The listing builds one solid part. Answer for the finished solid, in the listing's coordinates (mm). Face numbers are marked on the shaded views. A direction names the side the tool comes from. Give positions to 0.01 mm unless a question says otherwise; leave off trailing zeros. Write each loop counter-clockwise with the first axis right and the second up, starting at its lowest first coordinate (ties: lowest second). Pieces come first, ordered by that corner, then holes. Notation, with made-up numbers: (58.25, -26) - (104.25, -26) arc R37 cw to (104.25, 10) - close; hole circle Ø3 at (29.25, -22). An arc over 180 degrees is marked (long way). One line per question, with ' | ' between items. Start each with the question number.
1. A cutting plane is placed at D-D (x = -35). Determine the outline of the cut face in (y, z), then the cut area to 3 significant figures.
2. Given P1, Ø6, axis at x = 17, y = -1, coming from the +Z side; P2, Ø6, axis at x = -12, z = 6, coming from the +Y side; P3, Ø1, axis at y = 2, z = 4, coming from the +X side, each flat-ended and moving along its own axis, determine where each tip first touches the part or whether it passes through.
3. A cutting plane is placed at B-B (z = 9). Determine the outline of the cut face in (x, y), then the cut area to 3 significant figures.
4. A cutting plane is placed at C-C (x = 12). Determine the outline of the cut face in (y, z).
5. Find the intervals of material crossed by L1, parallel to Y at x = 0, z = 7.75; L2, parallel to X at y = -1.5, z = 1.5; L3, parallel to X at y = -0.5, z = 5.25, in increasing order. Write a range as from..to.
6. For the marked faces 1 and 2, determine the directions among +Z, -Z, +X, -X, +Y, -Y from which every point of the face is accessible in a straight line to the end or side of a thin tool.
7. A cutting plane is placed at A-A (x = 0). Determine the outline of the cut face in (y, z).
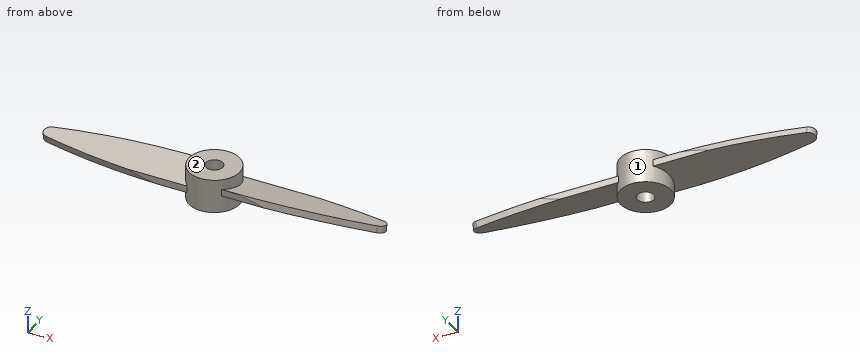
Autodesk Inventor part; units mm, degrees
ref_plane "Work Plane1" through (0, 7.5, 0) normal (0, 1, 0) x (-1, 0, 0)
ref_plane "Work Plane2" through (-7.5, 0, 0) normal (1, 0, 0) x (0, 1, 0)
ref_plane "Work Plane3" through (7.5, 0, 0) normal (1, 0, 0) x (0, 1, 0)
sketch "Sketch - Propeller Connecter" plane through (0, 0, 0) normal (0, 0, 1) x (1, 0, 0)
  circle A0 centre (0, 0) radius 7.5
  circle A1 centre (0, 0) radius 2.5
  dimension "d0" = 15
  dimension "d1" = 5
extrude "Extrusion1" add sketch "Sketch - Propeller Connecter" along normal blind 10
ref_plane "Work Plane1" through (0, 7.5, 0) normal (0, 1, 0) x (-1, 0, 0)
ref_plane "Work Plane2" through (-7.5, 0, 0) normal (1, 0, 0) x (0, 1, 0)
sketch "Sketch3" plane through (-7.5, 0, 0) normal (1, 0, 0) x (0, 1, 0)
  line L0 (7.5, 10) -> (-7.5, 10)
  line L1 (7.5, 10) -> (7.5, 0)
  line L2 (7.5, 0) -> (7.5, 10)
  line L3 (-7.5, 0) -> (7.5, 0)
  line L4 (-7.5, 10) -> (-7.5, 0)
  line L5 (-7.5, 0) -> (-7.5, 10)
  line L6 (5.5, 7) -> (-5.5, 5)
  line L7 (5.5, 5) -> (-5.5, 3)
  line L8 (5.5, 5) -> (5.5, 7)
  line L9 (-5.5, 3) -> (-5.5, 5)
  point P0 (0, 0)
  point P1 (0, 5)
  dimension "d27" = 5
  dimension "d28" = 3
  dimension "d29" = 3
  dimension "d30" = 5
  dimension "d32" = 2
  dimension "d33" = 2
  dimension "d34" = 2
  dimension "d35" = 2
sketch3d "3D Sketch2"
ref_plane "Work Plane3" through (7.5, 0, 0) normal (1, 0, 0) x (0, 1, 0)
sketch "Sketch4" plane through (7.5, 0, 0) normal (1, 0, 0) x (0, 1, 0)
  line L0 (5.5, 5) -> (-5.5, 7)
  line L1 (5.5, 3) -> (-5.5, 5)
  line L2 (5.5, 3) -> (5.5, 5)
  line L3 (-5.5, 5) -> (-5.5, 7)
  line L4 (7.5, 10) -> (-7.5, 10)
  line L5 (-7.5, 0) -> (7.5, 0)
  line L6 (-7.5, 0) -> (-7.5, 10)
  line L7 (7.5, 0) -> (7.5, 10)
  point P0 (0, 0)
  point P1 (0, 5)
  dimension "d38" = 3
  dimension "d39" = 5
  dimension "d40" = 3
  dimension "d42" = 5
  dimension "d43" = 2
  dimension "d44" = 2
  dimension "d45" = 2
  dimension "d46" = 2
sketch3d "3D Sketch3"
extrude "Extrusion2" add sketch "Sketch4" against normal blind 5 contours L2 L1 L3 L0
extrude "Extrusion3" add sketch "Sketch4" along normal blind 50 contours L2 L1 L3 L0
extrude "Extrusion4" add sketch "Sketch3" along normal blind 5 contours L8 L7 L9 L6
extrude "Extrusion5" add sketch "Sketch3" against normal blind 50 contours L8 L7 L9 L6
sketch "Sketch8" plane through (-5.099, -5.5, 3) normal (0, 0.1788854, -0.9838699) x (-1, 0, 0)
  line L0 (52.401, 0) -> (0, 0)
  line L1 (52.401, 11.1803) -> (52.401, 0)
  arc A0 (2.3083, 0) -> (52.401, 5.5902) centre (5.3498, 199.9769) ccw
  line L2 (52.401, 5.5902) -> (52.401, 0)
  line L3 (52.401, 0) -> (8.3914, 0)
  point P0 (-5.099, 4.8746)
  dimension "d59" = 200
extrude "Extrusion6" cut sketch "Sketch8" against normal blind 30 contours L0 A0 L1
sketch "Sketch15" plane through (57.5, 5.5, 3) normal (0, -0.1788854, -0.9838699) x (-1, 0, 0)
  line L0 (52.401, -0.3578) -> (52.401, 0)
  arc A0 (52.401, 0) -> (-0.7421, -4.8746) centre (43.9347, -199.8207) ccw
  line L1 (-0.7421, -4.8746) -> (-0.7421, 0)
  line L2 (-0.7421, 0) -> (35.4685, 0)
  point P0 (57.5, -4.8746)
  dimension "d67" = 200
extrude "Extrusion7" cut sketch "Sketch15" against normal blind 30
sketch "Sketch16" plane through (-57.5, 5.5, 7) normal (0, -0.1788854, 0.9838699) x (1, 0, 0)
  line L0 (52.401, -0.3578) -> (52.401, 0)
  line L1 (0, -5.9479) -> (0, 0)
  arc A0 (52.401, 0) -> (0, -5.9479) centre (48.5604, -199.9631) ccw
  line L2 (0, 0) -> (44.7198, 0)
  line L3 (52.401, 0) -> (0, 0)
  point P0 (57.5, -6.6635)
  dimension "d70" = 200
extrude "Extrusion8" cut sketch "Sketch16" against normal blind 30 contours L1 L2 A0
sketch "Sketch17" plane through (5.099, -5.5, 7) normal (0, 0.1788854, 0.9838699) x (1, 0, 0)
  ellipse E0 centre (-5.099, 5.5902) end of major axis (-5.099, -2.0328) minor radius 7.5 (0, 0) -> (0, 11.1803) ccw
  line L0 (52.401, 6.8321) -> (52.401, 0)
  arc A0 (0, 0) -> (52.401, 6.8321) centre (0.5699, 199.9992) ccw
  line L1 (52.401, 0) -> (1.1398, 0)
  line L2 (0, 0) -> (52.401, 0)
  point P0 (-5.099, 6.6635)
  dimension "d73" = 200
extrude "Extrusion9" cut sketch "Sketch17" against normal blind 30
fillet "Fillet1" radius 2 1 edges at (57.5, 1.0459, 4.8098)
fillet "Fillet2" radius 2 1 edges at (-57.5, -0.176, 4.968)
properties part number "propeller"
Determined:
1) outline: (-4.39, 5.2) - (-4.03, 3.27) - (4.21, 4.77) - (3.86, 6.7) - close | area: 16.5 mm2
2) P1: z = 6.73 | P2: y = 5.5 | P3: x = 50.16
3) outline: circle Ø15 at (0, 0); hole circle Ø5 at (0, 0) | area: 157 mm2
4) outline: (-5.5, 5) - (5.5, 3) - (5.5, 5) - (-5.4, 6.98) - (-5.5, 6.44) - close
5) L1: -7.5..-2.5, 2.5..7.5 | L2: -7.35..-2, 2..7.35 | L3: -50.26..-2.45, 2.45..49.73
6) face 1: none | face 2: +Z, +X, -X, +Y, -Y
7) outline: (-7.5, 0) - (-2.5, 0) - (-2.5, 10) - (-7.5, 10) - close; (2.5, 0) - (7.5, 0) - (7.5, 10) - (2.5, 10) - close
